from build123d import *

# Parameters (mm, degrees)
SKETCH1_W          = 38.1
SKETCH1_H          = 4.7625
CHAMFER1_SIZE      = 0.79375
CUT_EXTRUDE2_DEPTH = 4.16052


with BuildPart() as part:
    # Sketch1 → Revolve1 (revolve)
    with BuildSketch(Plane(origin=(0, 0, 0), x_dir=(0, 0, -1), z_dir=(1, 0, 0)), mode=Mode.PRIVATE) as revolve1_sk:
        with Locations((19.05, 2.38125)):
            Rectangle(SKETCH1_W, SKETCH1_H)
    revolve(revolve1_sk.sketch.rotate(Axis((0, 0, -38.1), (0, 0, 1)), 180), axis=Axis((0, 0, -38.1), (0, 0, 1)))

    # Chamfer1
    chamfer1_edges = [part.edges().sort_by_distance(p)[0] for p in [
        (0, 4.7625, -38.1),
    ]]
    chamfer(chamfer1_edges, length=CHAMFER1_SIZE)

    # Sketch7 → Revolve2 (revolve)
    with BuildSketch(Plane(origin=(0, 0, 0), x_dir=(0, 0, -1), z_dir=(1, 0, 0)), mode=Mode.PRIVATE) as revolve2_sk:
        with BuildLine():
            Line((0, 9.9187), (0.29718, 9.9187))
            Line((0.29718, 9.9187), (5.9436, 5.010341978))
            ThreePointArc((5.9436, 5.010341978), (6.252633175, 4.826486559), (6.606483481, 4.7625))
            Line((6.606483481, 4.7625), (6.606483481, 0))
            Line((6.606483481, 0), (0, 0))
            Line((0, 0), (0, 9.9187))
        make_face()
    revolve(revolve2_sk.sketch.rotate(Axis((0, 0, 0), (0, 0, -1)), 180), axis=Axis((0, 0, 0), (0, 0, -1)))

    # Boss-Extrude1 cone 1 section (through the dimple's axis) → Boss-Extrude1 (revolve)
    with BuildSketch(Plane(origin=(0, 0, -6.606483481), x_dir=(0, -1, 0), z_dir=(1, 0, 0))):
        Polygon((0, 0), (4.7625, 0), (0, 4.59909279), align=None)
    revolve(axis=Axis((0, 0, -6.606483481), (0, 0, -1)))

    # Sketch5 → Cut-Extrude2 (cut)
    with BuildSketch(Plane.XY):
        Polygon((0, 3.207902433), (-2.778125, 1.603951217), (-2.778125, -1.603951217), (0, -3.207902433), (2.778125, -1.603951217), (2.778125, 1.603951217), align=None)
    extrude(amount=-CUT_EXTRUDE2_DEPTH, mode=Mode.SUBTRACT)

    # Cut-Extrude3 cone 1 section (through the dimple's axis) → Cut-Extrude3 (revolve, cut)
    with BuildSketch(Plane(origin=(0, 0, 0), x_dir=(0, -1, 0), z_dir=(1, 0, 0))):
        Polygon((0, 0), (3.207902433, 0), (0, 1.852083333), align=None)
    revolve(axis=Axis((0, 0, 0), (0, 0, -1)), mode=Mode.SUBTRACT)


solid = part.part
Read the model definition and answer for the solid it produces. Units are mm, in the model's axes. A direction names the side the tool comes from. Coordinates: 2 decimals unless noted, no trailing zeros. Loops run counter-clockwise (first coordinate to the right, second up) from the corner with the lowest first, then second, coordinate; pieces in that order, holes last. Notation, with made-up numbers: (17, 49) -> (57, 49) arc R34 ccw to (57, 79) -> close; hole circle Ø5 at (68.25, -19). An arc over 180 degrees is marked (long way). Write item = value, one per line. Start each with the question number.
1) The part is cut by section A-A, the plane y = 0. Determine the outline of the cut face in (x, z), plus the area to 3 significant figures.
2) The mould has two halves that part along Y. Classify faces 1 (the face through (1.4, 2.4, -2.1)), 2 (the face through (3.19, 4.17, -5.67)), 3 (the face through (0, 4, 0)): pulls with the +Y half, pulls with the -Y half, needs draft (parallel to the pull), parting line crosses it, or undercut.
3) The part is cut by section B-B, the plane z = -30. Determine the outline of the cut face in (x, y) (1 decimal), plus the area to 3 significant figures.
4) The part is cut by section C-C, the plane z = -5.5. Determine the outline of the cut face in (x, y).
5) Given P1, Ø1.6, axis at y = -0.5, z = -1.5, coming from the -X side; P2, Ø8, axis at y = 2, z = -19.5, coming from the +X side; P3, Ø1, axis at y = -0.5, z = -2.5, coming from the +X side, each flat-ended and moving along its own axis, determine where each tip first touches the part or whether it passes through.
6) For faces 4 (the face through (-4.65, 1.03, -22.17)), 5 (the face through (0, 0, -38.1)), 6 (the face through (1.4, -2.4, -2.1)), determine the directions among +Z, -Z, +X, -X, +Y, -Y from which every point of the face is accessible in a straight line to the end or side of a thin tool.
7) Find the intervals of material crossed by L1, parallel to Z at x = 0.25, y = -5; L2, parallel to X at y = -0.25, z = -2.5; L3, parallel to Z at x = -1.25, y = -0.5, in increasing order. Write a range as from..to.
Result:
q1.outline = (-9.92, -0.3) -> (-5.01, -5.94) arc R1.01 cw to (-4.76, -6.61) -> (-4.76, -37.31) -> (-3.97, -38.1) -> (3.97, -38.1) -> (4.76, -37.31) -> (4.76, -6.61) arc R1.01 cw to (5.01, -5.94) -> (9.92, -0.3) -> (9.92, 0) -> (3.21, 0) -> (2.78, -0.25) -> (2.78, -4.16) -> (-2.78, -4.16) -> (-2.78, -0.25) -> (-3.21, 0) -> (-9.92, 0) -> close
q1.area = 373 mm²
q2.face_1 = undercut
q2.face_2 = parting line crosses it
q2.face_3 = needs draft
q3.outline = circle Ø9.5 at (0, 0)
q3.area = 71.3 mm²
q4.outline = circle Ø10.79 at (0, 0)
q5.P1 = -9.56
q5.P2 = 4.76
q5.P3 = 8.42
q6.face_4 = -Z
q6.face_5 = -Z, +X, -X, +Y, -Y
q6.face_6 = +Z
q7.L1 = -5.95..0
q7.L2 = -8..-2.78, 2.78..8
q7.L3 = -38.1..-4.16
